Verification items for the finished model (mm, model axes). A direction names the side the tool comes from. Coordinates: 2 decimals unless noted, no trailing zeros. Order: outer loops, then holes, each group sorted by start corner. A loop starts at its lowest first (then second) coordinate and runs counter-clockwise, first axis right, second up. Notation, with made-up numbers: (36.5, -5) -> (66.5, -5) arc R15 ccw to (66.5, 22) -> close; hole circle Ø1 at (26, 53.5). An arc over 180 degrees is marked (long way). Answer as CSV lines item,"result".
```python
from build123d import *

# Parameters (mm, degrees)
SKETCH1_W           = 190.5
SKETCH1_H           = 6.35
BOSS_EXTRUDE1_DEPTH = 101.6
CUT_EXTRUDE1_DEPTH  = 216.993362167
SKETCH3_W           = 50.8
SKETCH3_H           = 50.8
BOSS_EXTRUDE2_DEPTH = 6.35
FILLET1_R           = 25.4
SKETCH4_W           = 54.356
SKETCH4_H           = 6.35
BOSS_EXTRUDE3_DEPTH = 114.9016


with BuildPart() as part:
    # Sketch1 → Boss-Extrude1 (new body)
    with BuildSketch(Plane(origin=(0, 0, 0), x_dir=(1, 0, 0), z_dir=(0, 1, 0))):
        with Locations((95.25, 3.175)):
            Rectangle(SKETCH1_W, SKETCH1_H)
    extrude(amount=BOSS_EXTRUDE1_DEPTH)

    # Sketch2 → Cut-Extrude1 (cut, through all)
    with BuildSketch(Plane(origin=(0, 0, -6.35), x_dir=(-1, 0, 0), z_dir=(0, 0, -1))):
        with BuildLine():
            Line((-177.8, 71.755), (-12.7, 71.755))
            ThreePointArc((-12.7, 71.755), (-10.795, 69.85), (-12.7, 67.945))
            Line((-12.7, 67.945), (-177.8, 67.945))
            ThreePointArc((-177.8, 67.945), (-179.705, 69.85), (-177.8, 71.755))
        make_face()
        with BuildLine():
            Line((-177.8, 33.655), (-12.7, 33.655))
            ThreePointArc((-12.7, 33.655), (-10.795, 31.75), (-12.7, 29.845))
            Line((-12.7, 29.845), (-177.8, 29.845))
            ThreePointArc((-177.8, 29.845), (-179.705, 31.75), (-177.8, 33.655))
        make_face()
    extrude(amount=-CUT_EXTRUDE1_DEPTH, mode=Mode.SUBTRACT)

    # Sketch3 → Boss-Extrude2 (add)
    with BuildSketch(Plane.XY):
        with Locations((25.4, -25.4)):
            Rectangle(SKETCH3_W, SKETCH3_H)
        with Locations((165.1, -25.4)):
            Rectangle(SKETCH3_W, SKETCH3_H)
    extrude(amount=-BOSS_EXTRUDE2_DEPTH)

    # Fillet1
    fillet1_edges = [part.edges().sort_by_distance(p)[0] for p in [
        (139.7, -50.8, -3.175),
        (0, -50.8, -3.175),
        (50.8, -50.8, -3.175),
        (190.5, -50.8, -3.175),
    ]]
    fillet(fillet1_edges, radius=FILLET1_R - 0.0001)  # a hair under: the kernel refuses the full size

    # Sketch4 → Boss-Extrude3 (add)
    with BuildSketch(Plane.XZ):
        with Locations((95.25, -3.175)):
            Rectangle(SKETCH4_W, SKETCH4_H)
    extrude(amount=BOSS_EXTRUDE3_DEPTH)


solid = part.part
```
Item 1: Section check C-C, the plane y = -43. Record the boundary of the cut face in (x, z).
Answer list:
outline,"(7.09, -6.35) -> (43.71, -6.35) -> (43.71, 0) -> (7.09, 0) -> close; (68.07, -6.35) -> (122.43, -6.35) -> (122.43, 0) -> (68.07, 0) -> close; (146.79, -6.35) -> (183.41, -6.35) -> (183.41, 0) -> (146.79, 0) -> close"
Item 2: Thickness scan on line 1 (X direction, y = -12.5, z = -3.5); line 2 (Y direction, x = 51, z = -4.5) (3 decimals); line 3 (Y direction, x = 81.5, z = -0.5) (3 decimals). Record the ranges inside material, lowest first.
Answer list:
line 1,"0 to 50.8, 68.07 to 122.43, 139.7 to 190.5"
line 2,"0 to 29.845, 33.655 to 67.945, 71.755 to 101.6"
line 3,"-114.902 to 29.845, 33.655 to 67.945, 71.755 to 101.6"
Item 3: Tool access check on faces 4 (the flat face through (190.5, 37, -3)), 5 (the cylindrical face through (43.56, -43.16, -3.22)), 6 (the flat face through (94, 67.945, -3)). Record the directions out of +Z, -Z, +X, -X, +Y, -Y that give a thin tool (end or side, any length) a straight path to the whole face; none if there is none.
Answer list:
face 4,"+Z, -Z, +X, +Y, -Y"
face 5,"+Z, -Z, -Y"
face 6,"+Z, -Z"
Item 4: Section check B-B, the plane x = 57. Record the boundary of the cut face in (y, z) (3 decimals), plus the area to 3 significant figures.
Answer list:
outline,"(0, -6.35) -> (29.845, -6.35) -> (29.845, 0) -> (0, 0) -> close; (33.655, -6.35) -> (67.945, -6.35) -> (67.945, 0) -> (33.655, 0) -> close; (71.755, -6.35) -> (101.6, -6.35) -> (101.6, 0) -> (71.755, 0) -> close"
area,"597 mm2"
Item 5: Section check D-D, the plane y = -80. Record the boundary of the cut face in (x, z), plus the area to 3 significant figures.
Answer list:
outline,"(68.07, -6.35) -> (122.43, -6.35) -> (122.43, 0) -> (68.07, 0) -> close"
area,"345 mm2"
Item 6: Depth check by flat-ended pin: pin 1 Ø3 at (x, z) = (135, -4) entering from -Y; pin 2 Ø12 at (x, y) = (86, 69.5) entering from +Z; pin 3 Ø1 at (y, z) = (-79, -1) entering from -X; pin 4 Ø12 at (x, y) = (129, -45) entering from -Z. Enter the tip coordinate at first touch or a pass-through.
Answer list:
pin 1,"y = 0"
pin 2,"z = 0"
pin 3,"x = 68.07"
pin 4,"through"
Item 7: Section check A-A, the plane z = -2.75. Count the separate pieces of the cut face and the enclosed holes in it, plus the area to 3 significant figures.
Answer list:
separate pieces,"1"
enclosed holes,"2"
area,"28,900 mm2"
Item 8: Release check for a two-part mould opening along X. For faces 1 (the flat face through (94, 29.845, -3)), 2 (the flat face through (0, 37, -3)), 3 (the flat face through (95, -114.902, -3)) record: +X half, -X half, draft (parallel to the pull), parting line (faces both ways), or undercut.
Answer list:
face 1,"undercut"
face 2,"-X half"
face 3,"draft"
